```python
from build123d import *

# Parameters (mm, degrees)
RESSALTO_EXTRUS_O1_DEPTH   = 20
ESBO_O3_R                  = 3.075
CORTE_EXTRUS_O1_DEPTH      = 20
ESBO_O4_R                  = 5.25
CORTE_EXTRUS_O2_DEPTH      = 6
ESBO_O5_R                  = 3.075
CORTE_EXTRUS_O3_DEPTH      = 1
CORTE_EXTRUS_O3_DEPTH_BACK = 80
ESBO_O6_R                  = 5.25
CORTE_EXTRUS_O4_DEPTH      = 6
FILETE1_R                  = 0.5


with BuildPart() as part:
    # Esboço1 → Ressalto-extrusão1 (new body)
    with BuildSketch(Plane(origin=(0, 0, 0), x_dir=(1, 0, 0), z_dir=(0, 1, 0))):
        with BuildLine():
            Line((61.23724357, 60), (87.707972894, 60))
            ThreePointArc((87.707972894, 60), (89.475739847, 60.732233047), (90.207972894, 62.5))
            Line((90.207972894, 62.5), (90.207972894, 72.5))
            ThreePointArc((90.207972894, 72.5), (89.475739847, 74.267766953), (87.707972894, 75))
            Line((87.707972894, 75), (52.115256883, 75))
            ThreePointArc((52.115256883, 75), (48.223697971, 75.513600543), (44.598633294, 77.019230769))
            ThreePointArc((44.598633294, 77.019230769), (-32.102711223, 83.008529273), (-84.815301953, 26.96969697))
            ThreePointArc((-84.815301953, 26.96969697), (-88.441850634, 21.92835115), (-94.345111161, 20))
            Line((-94.345111161, 20), (-108.409715081, 20))
            ThreePointArc((-108.409715081, 20), (-109.823928643, 19.414213562), (-110.409715081, 18))
            Line((-110.409715081, 18), (-110.409715081, 12))
            ThreePointArc((-110.409715081, 12), (-109.823928643, 10.585786438), (-108.409715081, 10))
            Line((-108.409715081, 10), (-86.168439698, 10))
            ThreePointArc((-86.168439698, 10), (-84.855375369, 10.491403941), (-84.187556027, 11.724137931))
            ThreePointArc((-84.187556027, 11.724137931), (-27.432289416, 80.451659382), (59.487608039, 60.714285714))
            ThreePointArc((59.487608039, 60.714285714), (60.292332387, 60.185449751), (61.23724357, 60))
        make_face()
    extrude(amount=RESSALTO_EXTRUS_O1_DEPTH)

    # Esboço3 → Corte-extrusão1 (cut)
    with BuildSketch(Plane.XY.offset(-60)):
        with Locations((79.862425804, 9.799419725)):
            Circle(ESBO_O3_R)
    extrude(amount=-CORTE_EXTRUS_O1_DEPTH, mode=Mode.SUBTRACT)

    # Esboço4 → Corte-extrusão2 (cut)
    with BuildSketch(Plane(origin=(0, 0, -75), x_dir=(-1, 0, 0), z_dir=(0, 0, -1))):
        with Locations((-79.862425804, 9.799419725)):
            Circle(ESBO_O4_R)
    extrude(amount=-CORTE_EXTRUS_O2_DEPTH, mode=Mode.SUBTRACT)

    # Esboço5 → Corte-extrusão3 (cut, two sides)
    with BuildSketch(Plane.XY.offset(-10)) as corte_extrus_o3_sk:
        with Locations((-100.179715081, 10)):
            Circle(ESBO_O5_R)
    extrude(amount=CORTE_EXTRUS_O3_DEPTH, mode=Mode.SUBTRACT)
    extrude(corte_extrus_o3_sk.sketch, amount=-CORTE_EXTRUS_O3_DEPTH_BACK, mode=Mode.SUBTRACT)

    # Esboço6 → Corte-extrusão4 (cut)
    with BuildSketch(Plane(origin=(0, 0, -20), x_dir=(-1, 0, 0), z_dir=(0, 0, -1))):
        with Locations((100.179715081, 10)):
            Circle(ESBO_O6_R)
    extrude(amount=-CORTE_EXTRUS_O4_DEPTH, mode=Mode.SUBTRACT)

    # Filete1
    filete1_edges = [part.edges().sort_by_distance(p)[0] for p in [
        (-88.441850634, 20, -21.92835115),
        (69.911614889, 0, -75),
        (89.475739847, 0, -74.267766953),
        (90.207972894, 0, -67.5),
        (-101.377413121, 20, -20),
        (89.475739847, 0, -60.732233047),
        (74.472608232, 0, -60),
        (60.292332387, 0, -60.185449751),
        (-27.432289416, 0, -80.451659382),
        (-84.855375369, 0, -10.491403941),
        (-97.289077389, 0, -10),
        (-109.823928643, 0, -10.585786438),
        (-110.409715081, 0, -15),
        (-109.823928643, 0, -19.414213562),
        (-101.377413121, 0, -20),
        (-109.823928643, 20, -19.414213562),
        (-88.441850634, 0, -21.92835115),
        (-32.102711223, 0, -83.008529273),
        (48.223697971, 0, -75.513600543),
        (-110.409715081, 20, -15),
        (-109.823928643, 20, -10.585786438),
        (-97.289077389, 20, -10),
        (-84.855375369, 20, -10.491403941),
        (-27.432289416, 20, -80.451659382),
        (60.292332387, 20, -60.185449751),
        (74.472608232, 20, -60),
        (48.223697971, 20, -75.513600543),
        (89.475739847, 20, -60.732233047),
        (90.207972894, 20, -67.5),
        (89.475739847, 20, -74.267766953),
        (69.911614889, 20, -75),
        (-32.102711223, 20, -83.008529273),
    ]]
    fillet(filete1_edges, radius=FILETE1_R)


solid = part.part
```
Could you check a few things on this model? Use its own coordinates, in mm. A direction names the side the tool comes from. Give positions to 0.01 mm unless a question says otherwise; leave off trailing zeros. Write each loop counter-clockwise with the first axis right and the second up, starting at its lowest first coordinate (ties: lowest second). Pieces come first, ordered by that corner, then holes. Notation, with made-up numbers: (85, 35) -> (142, 35) arc R26 cw to (142, 57) -> close; hole circle Ø2 at (77.5, -9.75). An arc over 180 degrees is marked (long way). Write each question's results on one line, items separated by ' | '.
1. If we mould it in two halves opening along X, with no side actions, what happens to faces 1 (the cylindrical face through (-28.67, 9.87, -80.02)), 2 (the flat face through (74, 10, -60)), 3 (the cylindrical face through (-31.061, 9.867, -83.404))? For each: released by +X, released by -X, zero draft, split by the parting line, or undercut.
Check sheet entries:
face 1: undercut | face 2: zero draft | face 3: split by the parting line
2. I need wall thicknesses on L1, parallel to X at y = 8.75, z = -67.5; L2, parallel to Z at x = 77, y = 13.75; L3, parallel to X at y = 9.25, z = -17.5. Which ranges of each line are inside material? Lowest first, please.
Check sheet entries:
L1: x = -58.01 to -51.66, 51.66 to 76.97, 82.75 to 90.21 | L2: z = -69 to -60 | L3: x = -110.41 to -105.38, -94.98 to -83.18
3. I want a section at A-A, the plane y = 2.5. Write out the boundary of the cut face in (x, z), then the cut area to 3 significant figures.
Check sheet entries:
outline: (-110.41, -18) arc R2 ccw to (-108.41, -20) -> (-94.35, -20) arc R10 cw to (-84.82, -26.97) arc R89 ccw to (44.6, -77.02) arc R15 cw to (52.12, -75) -> (87.71, -75) arc R2.5 ccw to (90.21, -72.5) -> (90.21, -62.5) arc R2.5 ccw to (87.71, -60) -> (61.24, -60) arc R2.5 ccw to (59.49, -60.71) arc R85 cw to (-84.19, -11.72) arc R2 ccw to (-86.17, -10) -> (-108.41, -10) arc R2 ccw to (-110.41, -12) -> close | area: 1,510 mm²
4. Will these pins go through, and if not, where does the flat tip stop? pin 1 Ø11.5 at (x, y) = (-99.5, 11) entering from -Z; pin 2 Ø5 at (x, y) = (79, 7) entering from -Z; pin 3 Ø1 at (y, z) = (3.5, -52.5) entering from -X.
Check sheet entries:
pin 1: stops at z = -20.02 | pin 2: stops at z = -75 | pin 3: stops at x = -72.23
5. On a 3-axis mill with a long thin cutter (end or side, diameter ignored), from which of +Z, -Z, +X, -X, +Y, -Y can I reach the whole of each face in a straight line? I mean faces 4 (the flat face through (-100.1, 6.6, -14)), 5 (the flat face through (70, 10, -75)), 6 (the flat face through (-110.41, 10, -15)), 7 (the flat face through (-106, 10, -20)), 8 (the flat face through (4, 20, -87)). Say none if no direction works.
Check sheet entries:
face 4: -Z | face 5: -Z, +X, +Y, -Y | face 6: +Z, -Z, -X, +Y, -Y | face 7: -Z, -X, +Y, -Y | face 8: +Z, -Z, +X, -X, +Y
